Answer from the drawing. Dimensions are ordinates in mm from the lowest x, y and z of the part. A direction names the side the tool comes from. Round coordinates to 2 decimals unless told otherwise and drop trailing zeros. Loops run counter-clockwise (first coordinate to the right, second up) from the corner with the lowest first, then second, coordinate; pieces in that order, holes last. Notation, with made-up numbers: M 83.25,53.25 L 106.25,53.25 A27 ccw 106.25,90.25 Z; hole C -10.75,-34 d11. An arc over 180 degrees is marked long. Answer as a JSON object with one key per item and string values.
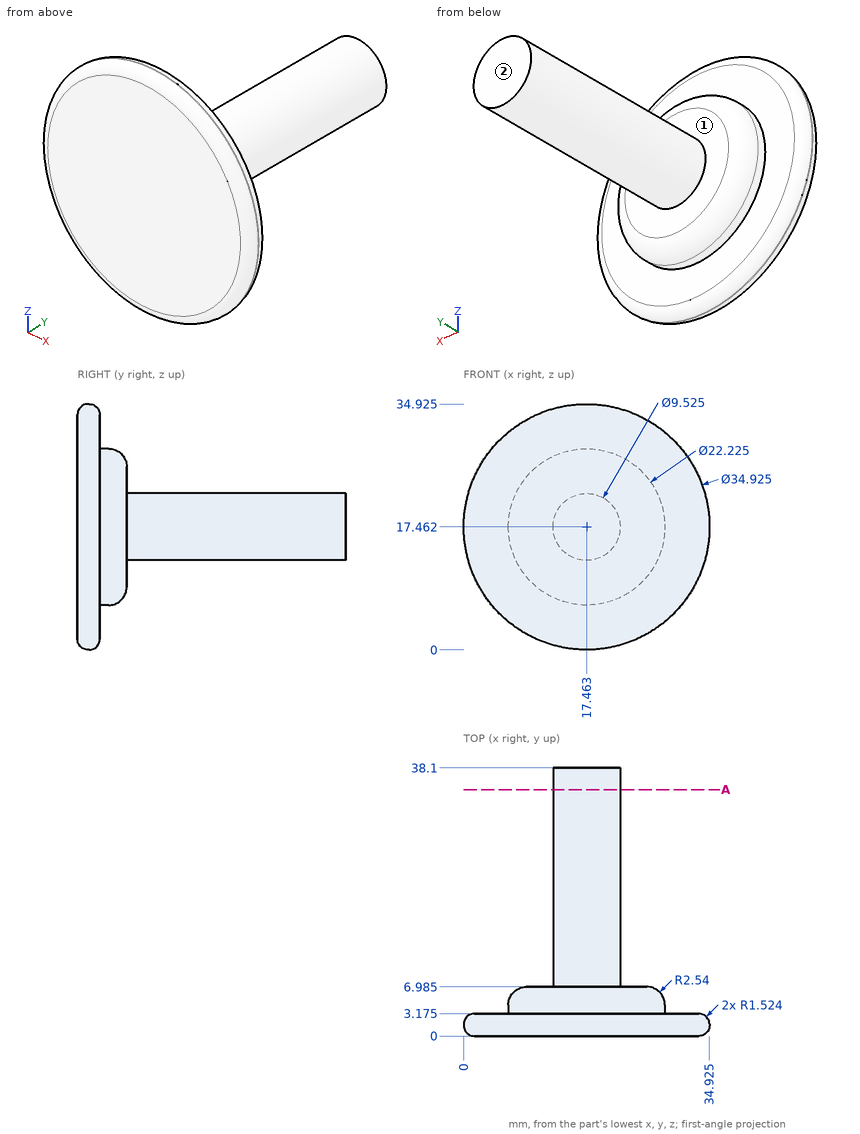
Item 1: Straight lines are drawn through the part: line 1 (Z direction, x = 17.5, y = 17.5) (1 decimal); line 2 (Y direction, x = 11.5, z = 16) (1 decimal); line 3 (Y direction, x = 16, z = 4.5) (1 decimal). For each, find the intervals that lie inside material, in ascending order.
Values follow:
{"line 1": "12.7 to 22.2", "line 2": "0 to 7", "line 3": "0 to 3.2"}
Item 2: Flat-ended cylindrical pins translate along their axes: P1, Ø6, axis at y = 23, z = 16.5, coming from the +X side (1 decimal); P2, Ø1, axis at x = 15, y = 20.5, coming from the -Z side; P3, Ø2, axis at y = 15.5, z = 13, coming from the -X side; P4, Ø3, axis at y = 6, z = 3.5, coming from the -X side. Find the tip coordinate at first contact, or state that the pin passes through.
Values follow:
{"P1": "x = 22.2", "P2": "z = 13.12", "P3": "x = 14.19", "P4": "through"}
Item 3: The part is cut by section A-A (y = 35). Give the vertices of the cut face in (x, z) (1 decimal).
Values follow:
{"outline": "C 17.5,17.5 d9.5"}
Item 4: Which of the six approach directions +Z, -Z, +X, -X, +Y, -Y give full straight-line access (tool end or side, diameter ignored) to the marked faces 1 and 2?
Values follow:
{"face 1": "+Y", "face 2": "+Z, -Z, +X, -X, +Y"}
